```python
from build123d import *

# Parameters (mm, degrees)
F0_W     = 42
F0_H     = 72
F0_W_2   = 36
F0_H_2   = 66
F1_DEPTH = 10
F2_R     = 3
F3_R     = 3
F5_D     = 10
F5_DEPTH = 3


with BuildPart() as f1:
    # F0 (on Front) → F1 (new body, symmetric)
    with BuildSketch(Plane.XZ):
        Rectangle(F0_W, F0_H)
        Rectangle(F0_W_2, F0_H_2, mode=Mode.SUBTRACT)
    extrude(amount=F1_DEPTH, both=True)

    # F2
    f2_edges = [f1.edges().sort_by_distance(p)[0] for p in [
        (21, 0, 36),
        (-21, 0, 36),
    ]]
    fillet(f2_edges, radius=F2_R)

    # F3
    f3_edges = [f1.edges().sort_by_distance(p)[0] for p in [
        (21, 0, -36),
        (-21, 0, -36),
    ]]
    fillet(f3_edges, radius=F3_R)

    # F5
    with Locations(Plane.YZ.offset(21)):
        with Locations((0, 18)):
            Hole(F5_D / 2, depth=F5_DEPTH)


solid = f1.part
```
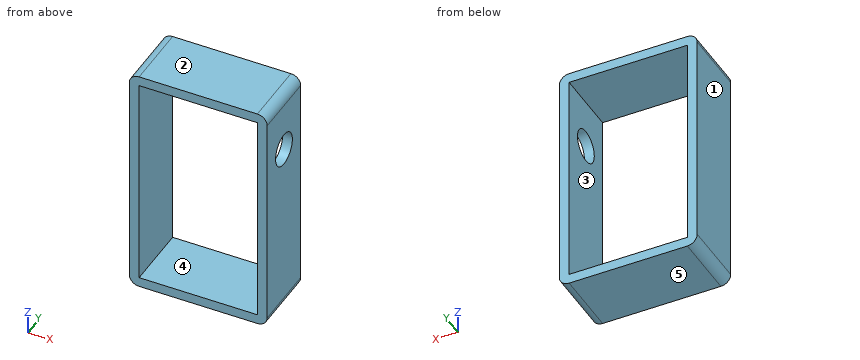
Read the model definition and answer for the solid it produces. Units are mm, in the model's axes. Face numbers are marked on the shaded views. A direction names the side the tool comes from. Give positions to 0.01 mm unless a question says otherwise; leave off trailing zeros. Order: outer loops, then holes, each group sorted by start corner. A loop starts at its lowest first (then second) coordinate and runs counter-clockwise, first axis right, second up.
(1) Find section A-A (x = -15). Give the vertices of the cut face in (y, z).
(2) Straight lines are drawn through the part: L1, parallel to Z at x = -16, y = 0.5; L2, parallel to X at y = -5.5, z = -15; L3, parallel to X at y = -2, z = 19. For each, find the intervals that lie inside material, in ascending order.
(3) Given pin 1 (6 mm diameter, centred on x = -16.5, z = -16.5, fed in from -Y); pin 2 (12 mm diameter, centred on x = -10, z = 17, fed in from -Y), each flat-ended and moving along its own axis, determine where each tip first touches the part or whether it passes through.
(4) Find section B-B (z = 18). Give the vertices of the cut face in (x, y), plus the area to 3 significant figures.
(5) For a pull along X with two mould halves and no side action, classify the marked faces 1, 2 and 3 as released by +X, released by -X, zero draft, split by the parting line, or undercut.
(6) For the marked faces 4 and 5, determine the directions among +Z, -Z, +X, -X, +Y, -Y from which every point of the face is accessible in a straight line to the end or side of a thin tool.
(7) Find section C-C (y = -8.5). Give the vertices of the cut face in (x, z).
(8) Find section D-D (z = 5). Give the vertices of the cut face in (x, y), plus the area to 3 significant figures.
Result sheet:
1. outline: (-10, -36) - (10, -36) - (10, -33) - (-10, -33) - close; (-10, 33) - (10, 33) - (10, 36) - (-10, 36) - close
2. L1: z = -36 to -33, 33 to 36
2. L2: x = -21 to -18, 18 to 21
2. L3: x = -21 to -18
3. pin 1: stops at y = -10
3. pin 2: passes through
4. outline: (-21, -10) - (-18, -10) - (-18, 10) - (-21, 10) - close; (18, -10) - (21, -10) - (21, -5) - (18, -5) - close; (18, 5) - (21, 5) - (21, 10) - (18, 10) - close
4. area: 90.0 mm2
5. face 1: released by -X
5. face 2: zero draft
5. face 3: undercut
6. face 4: +Y, -Y
6. face 5: -Z, +X, -X, +Y, -Y
7. outline: (-21, -33) arc R3 ccw to (-18, -36) - (18, -36) arc R3 ccw to (21, -33) - (21, 33) arc R3 ccw to (18, 36) - (-18, 36) arc R3 ccw to (-21, 33) - close; hole (-18, -33) - (18, -33) - (18, 33) - (-18, 33) - close
8. outline: (-21, -10) - (-18, -10) - (-18, 10) - (-21, 10) - close; (18, -10) - (21, -10) - (21, 10) - (18, 10) - close
8. area: 120 mm2
